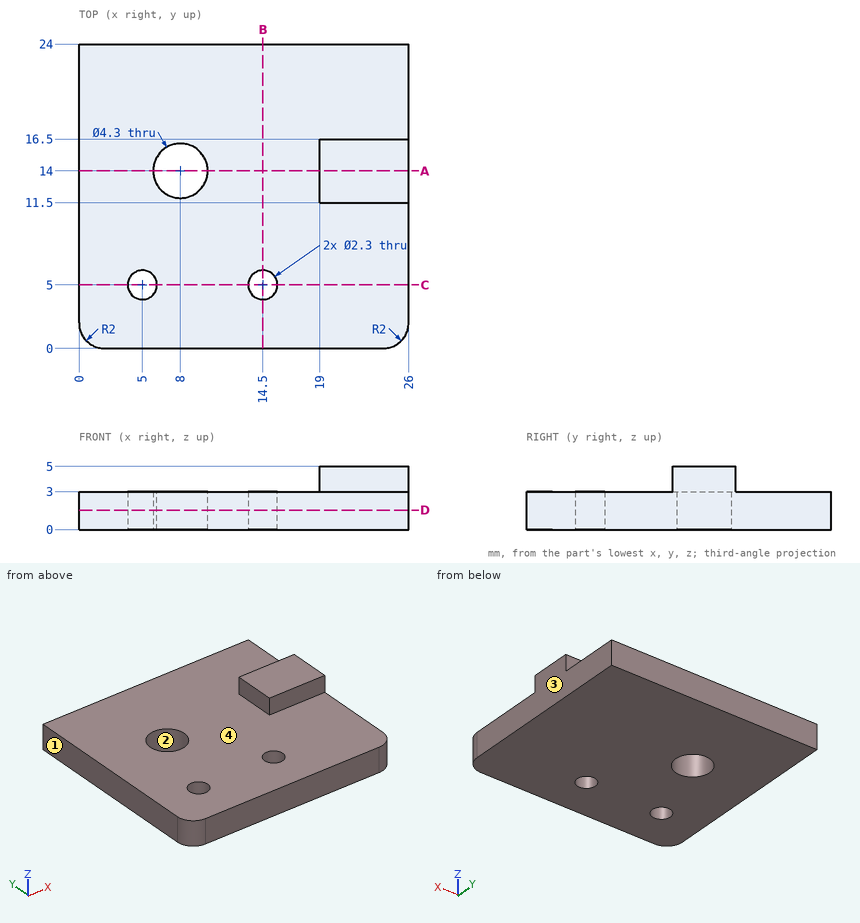
Geometry check sheet. Reference: drawing and pictorial views, mm from the part's lowest x, y, z. Give positions to 0.01 mm unless a question says otherwise; leave off trailing zeros. Write each loop counter-clockwise with the first axis right and the second up, starting at its lowest first coordinate (ties: lowest second). Pieces come first, ordered by that corner, then holes. Notation, with made-up numbers: M -22.75,34 L 0.25,34 A31 ccw 0.25,60 Z; hole C -27.5,33 d4. An arc over 180 degrees is marked long. Put each result on its own line as item: value. Start each with the question number.
1. Scan lines: line 1 along Y through (x, z) = (5, 0.75); line 2 along X through (y, z) = (4.5, 2.2); line 3 along Y through (x, z) = (8, 2). Record each from-to range of solid material in increasing order. Write a range as [from, to].
2. Section check B-B (x = 14.5). Record the cut outline in (y, z), and give its area (3 significant figures).
3. Section check D-D (z = 1.55). Record the cut outline in (x, y).
4. Section check C-C (y = 5). Record the cut outline in (x, z).
5. Go/stop test with flat-tipped pins: pin 1 Ø1 at (y, z) = (14, 4.5) entering from -X; pin 2 Ø1 at (x, y) = (14, 9) entering from +Z; pin 3 Ø4 at (x, y) = (8, 14) entering from +Z. Record where each tip stops, or that it passes through.
6. Section check A-A (y = 14). Record the cut outline in (x, z).
7. Draft check along X on the marked faces 1, 2, 3 and 4. Enter one of: +X half, -X half, draft (parallel to the pull), parting line (faces both ways), or undercut.
Answer list:
1. line 1: [0, 3.85], [6.15, 24]
1. line 2: [0, 3.96], [6.04, 13.46], [15.54, 26]
1. line 3: [0, 11.85], [16.15, 24]
2. outline: M 0,0 L 3.85,0 L 3.85,3 L 0,3 Z; M 6.15,0 L 24,0 L 24,3 L 6.15,3 Z
2. area: 65.1 mm2
3. outline: M 0,2 A2 ccw 2,0 L 24,0 A2 ccw 26,2 L 26,24 L 0,24 Z; hole C 5,5 d2.3; hole C 8,14 d4.3; hole C 14.5,5 d2.3
4. outline: M 0,0 L 3.85,0 L 3.85,3 L 0,3 Z; M 6.15,0 L 13.35,0 L 13.35,3 L 6.15,3 Z; M 15.65,0 L 26,0 L 26,3 L 15.65,3 Z
5. pin 1: x = 19
5. pin 2: z = 3
5. pin 3: through
6. outline: M 0,0 L 5.85,0 L 5.85,3 L 0,3 Z; M 10.15,0 L 26,0 L 26,5 L 19,5 L 19,3 L 10.15,3 Z
7. face 1: -X half
7. face 2: undercut
7. face 3: +X half
7. face 4: draft
